```python
from build123d import *

# Parameters (mm, degrees)
SKETCH1_R            = 1.091149581
SKETCH1_R_2          = 1.265238112
SKETCH1_R_3          = 1.717110749
SKETCH1_R_4          = 1.455402606
BOSS_EXTRUDE1_DEPTH  = 3.175
M4_CLEARANCE_HOLE1_D = 4.8


with BuildPart() as part:
    # Sketch1 → Boss-Extrude1 (new body)
    with BuildSketch(Plane.XY):
        Polygon((11.503555024, -3.77372269), (36.903555024, -3.77372269), (36.903555024, 57.275941722), (73.723553593, 57.275941722), (73.723553593, -3.77372269), (99.123553593, -3.77372269), (99.123553593, 66.34627731), (73.723553593, 66.34627731), (36.903555024, 66.34627731), (11.503555024, 66.34627731), align=None)
        with Locations((24.203555024, 53.64627731)):
            Circle(SKETCH1_R, mode=Mode.SUBTRACT)
        with Locations((24.203555024, 8.92627731)):
            Circle(SKETCH1_R_2, mode=Mode.SUBTRACT)
        with Locations((86.423553593, 53.64627731)):
            Circle(SKETCH1_R_3, mode=Mode.SUBTRACT)
        with Locations((86.423553593, 8.92627731)):
            Circle(SKETCH1_R_4, mode=Mode.SUBTRACT)
    extrude(amount=BOSS_EXTRUDE1_DEPTH)

    # M4 Clearance Hole1 (through all)
    with Locations(Plane.XY.offset(3.175)):
        with Locations((24.203555024, 53.64627731), (24.203555024, 8.92627731), (86.423553593, 8.92627731), (86.423553593, 53.64627731)):
            Hole(M4_CLEARANCE_HOLE1_D / 2)


solid = part.part
```
For this review, take the finished solid that the model builds, in its own axes (mm). A direction names the side the tool comes from. Round coordinates to 2 decimals unless told otherwise and drop trailing zeros. Write each loop counter-clockwise with the first axis right and the second up, starting at its lowest first coordinate (ties: lowest second). Pieces come first, ordered by that corner, then holes. Notation, with made-up numbers: (64.5, -27) - (113.5, -27) arc R20 ccw to (113.5, -7) - close; hole circle Ø7 at (55.25, -5). An arc over 180 degrees is marked (long way). Write each question's results on one line, items separated by ' | '.
Item 1: Take a section at B-B on z = 0.55. State the section outline as (x, y) points.
Calculated:
outline: (11.5, -3.77) - (36.9, -3.77) - (36.9, 57.28) - (73.72, 57.28) - (73.72, -3.77) - (99.12, -3.77) - (99.12, 66.35) - (11.5, 66.35) - close; hole circle Ø4.8 at (24.2, 8.93); hole circle Ø4.8 at (24.2, 53.65); hole circle Ø4.8 at (86.42, 8.93); hole circle Ø4.8 at (86.42, 53.65)
Item 2: To check wall thickness, follow line 1 along X through (y, z) = (8.5, 2.55); line 2 along X through (y, z) = (16, 2.1); line 3 along Y through (x, z) = (86, 1.95). State the ranges of each line that lie inside material, in increasing order. Write a range as from..to.
Calculated:
line 1: x = 11.5..21.84, 26.57..36.9, 73.72..84.06, 88.79..99.12 | line 2: x = 11.5..36.9, 73.72..99.12 | line 3: y = -3.77..6.56, 11.29..51.28, 56.01..66.35
Item 3: For faces 4 (the face through (86.736, 56.026, 1.565)), 5 (the face through (73.724, 27, 2)), list the 3-axis set-ups (+Z, -Z, +X, -X, +Y, -Y) from which the entire face can be reached by the end or side of a thin tool; tool diameter is ignored.
Calculated:
face 4: +Z, -Z | face 5: +Z, -Z, -Y
Item 4: Take a section at A-A on y = 19.5. State the section outline as (x, z) points (3 decimals).
Calculated:
outline: (11.504, 0) - (36.904, 0) - (36.904, 3.175) - (11.504, 3.175) - close; (73.724, 0) - (99.124, 0) - (99.124, 3.175) - (73.724, 3.175) - close
Item 5: For pin 1 (4 mm diameter, centred on x = 86.42, y = 8.93, fed in from -Z), flat-tipped, find the tip position at first contact; note if it passes through.
Calculated:
pin 1: passes through
Item 6: Draft analysis for pull direction Y (two halves, no side actions). For faces 1 (the face through (26.11, 7.47, 1.57)), 2 (the face through (99.124, 31, 2)), 3 (the face through (55, 57.276, 2)), state which applies: pulls with the +Y half, pulls with the -Y half, needs draft (parallel to the pull), parting line crosses it, or undercut.
Calculated:
face 1: undercut | face 2: needs draft | face 3: pulls with the -Y half
Item 7: Take a section at C-C on x = 57. State the section outline as (y, z) points (3 decimals).
Calculated:
outline: (57.276, 0) - (66.346, 0) - (66.346, 3.175) - (57.276, 3.175) - close
